Autodesk Inventor part; units mm, degrees
ref_plane "YZ Plane" through (0, 0, 0) normal (1, 0, 0) x (0, 1, 0)
ref_plane "XZ Plane" through (0, 0, 0) normal (0, 1, 0) x (-1, 0, 0)
ref_plane "XY Plane" through (0, 0, 0) normal (0, 0, 1) x (1, 0, 0)
sketch "Эскиз1" plane through (0, 0, 0) normal (0, 1, 0) x (-1, 0, 0)
  circle A0 centre (0, 0) radius 14
  arc A1 (-20.1, -12.4624) -> (-20.1, 12.4624) centre (0, 0) ccw
  line L0 (-20.1, 12.4624) -> (-20.1, -12.4624)
  line L1 (-20.1, 0) -> (21.15, 0)
  circle A2 centre (21.15, 0) radius 1.05
  circle A3 centre (12.8753, 16.7794) radius 1.05
  circle A4 centre (-5.474, 20.4293) radius 1.05
  circle A5 centre (12.8753, -16.7794) radius 1.05
  circle A6 centre (-5.474, -20.4293) radius 1.05
  dimension "d0" = 28
  dimension "d1" = 47.3
  dimension "d3" = 2.1
  dimension "d4" = 21.15
  dimension "d11" = 20.1
  dimension "d24" = 105
  dimension "d28" = 105
extrude "Выдавливание3" add sketch "Эскиз1" along normal blind 3
properties part number "держалка подша"
Input: part model. Units: mm. Frame: model coordinates. Give positions to 0.01 mm unless a question says otherwise; leave off trailing zeros. Loops run counter-clockwise (first coordinate to the right, second up) from the corner with the lowest first, then second, coordinate; pieces in that order, holes last. Notation, with made-up numbers: (-37, -25) - (-25, -25) arc R21 ccw to (-25, 2) - close; hole circle Ø5 at (6.25, 66). An arc over 180 degrees is marked (long way). Use CSV: the item, a comma, the result in double quotes. Start each with the question number.
Item 1: Line query: line 1 (X direction, y = 2.35, z = -0.5); line 2 (Z direction, x = 5, y = 1.6); line 3 (Z direction, x = -9.5, y = 1.05). Output: solid intervals per line, ascending.
Item 2: Mould query, pull axis X, two halves, no side actions, for faces 1 (the cylindrical face through (-23.634, 1.479, 0.856)), 2 (the cylindrical face through (5.702, 1.479, 21.454)), 3 (the flat face through (-11, 3, -10)), 4 (the cylindrical face through (-20.1, 1.5, 0)). Classes: pulls with the +X half, pulls with the -X half, needs draft (parallel to the pull), parting line crosses it, or undercut.
Item 3: Section C-C on y = 1. Return loops of the section in (x, z), then the cut area to 3 significant figures.
Item 4: Section D-D on z = 11. Return loops of the section in (x, y).
Item 5: Section B-B on z = 0. Return loops of the section in (x, y).
Item 6: Section A-A on x = 0. Return loops of the section in (y, z).
Ans:
1,line 1,"x = -23.64 to -22.07, -20.23 to -13.99, 13.99 to 20.1"
1,line 2,"z = -23.12 to -21.37, -19.49 to -13.08, 13.08 to 19.49, 21.37 to 23.12"
1,line 3,"z = -21.66 to -10.28, 10.28 to 21.66"
2,face 1,"parting line crosses it"
2,face 2,"undercut"
2,face 3,"needs draft"
2,face 4,"undercut"
3,outline,"(20.1, -12.46) - (20.1, 12.46) arc R23.65 ccw (long way) to start; hole circle Ø2.1 at (-21.15, 0); hole circle Ø28 at (0, 0); hole circle Ø2.1 at (-12.88, -16.78); hole circle Ø2.1 at (-12.88, 16.78); hole circle Ø2.1 at (5.47, -20.43); hole circle Ø2.1 at (5.47, 20.43)"
3,area,"1,060 mm2"
4,outline,"(-20.94, 0) - (-8.66, 0) - (-8.66, 3) - (-20.94, 3) - close; (8.66, 0) - (20.1, 0) - (20.1, 3) - (8.66, 3) - close"
5,outline,"(-23.65, 0) - (-22.2, 0) - (-22.2, 3) - (-23.65, 3) - close; (-20.1, 0) - (-14, 0) - (-14, 3) - (-20.1, 3) - close; (14, 0) - (20.1, 0) - (20.1, 3) - (14, 3) - close"
6,outline,"(0, -23.65) - (3, -23.65) - (3, -14) - (0, -14) - close; (0, 14) - (3, 14) - (3, 23.65) - (0, 23.65) - close"
